Build history of the part. All positions in model axes, mm. A direction names the side the tool comes from. Coordinates: 2 decimals unless noted, no trailing zeros. Order: outer loops, then holes, each group sorted by start corner. A loop starts at its lowest first (then second) coordinate and runs counter-clockwise, first axis right, second up. Notation, with made-up numbers: (-6, 6) - (4, 6) arc R26 ccw to (4, 37) - close; hole circle Ø4 at (-3, 41.5). An arc over 180 degrees is marked (long way). One line per item, written item: value.
from build123d import *

# Parameters (mm, degrees)
SKETCH_1_W          = 13.1
SKETCH_1_H          = 9.245579741
SKETCH_1_R          = 1
EXTRUDE_1_DEPTH     = 1.3
SKETCH_2_W          = 1.5
SKETCH_2_H          = 5
EXTRUDE_2_DEPTH     = 8
SKETCH_4_R          = 1
CUT_EXTRUDE_1_DEPTH = 15


with BuildPart() as part:
    # 草图1 → 凸台-拉伸1 (new body)
    with BuildSketch(Plane.XY):
        with Locations((6.55, 4.622789871)):
            Rectangle(SKETCH_1_W, SKETCH_1_H)
        with Locations((6.55, 7.245579741)):
            Circle(SKETCH_1_R, mode=Mode.SUBTRACT)
    extrude(amount=EXTRUDE_1_DEPTH)

    # 草图2 → 凸台-拉伸2 (add)
    with BuildSketch(Plane.XY.offset(1.3)):
        with Locations((0.75, 2.5)):
            Rectangle(SKETCH_2_W, SKETCH_2_H)
        with Locations((12.35, 2.5)):
            Rectangle(SKETCH_2_W, SKETCH_2_H)
    extrude(amount=EXTRUDE_2_DEPTH)

    # 草图4 → 切除-拉伸1 (cut)
    with BuildSketch(Plane.ZY):
        with Locations((7.3, 2.5)):
            Circle(SKETCH_4_R)
    extrude(amount=-CUT_EXTRUDE_1_DEPTH, mode=Mode.SUBTRACT)


solid = part.part
1. 3-axis set-ups, long thin cutter, end or side, ignore diameter. For faces 4 (the face through (0, 3, 5)), 5 (the face through (1.5, 2, 5)), 6 (the face through (1, 5, 5)): which of +Z, -Z, +X, -X, +Y, -Y reach the whole face in a straight line?
Values found:
face 4: +Z, -Z, -X, +Y, -Y
face 5: +Z, +Y, -Y
face 6: +Z, +X, -X, +Y
2. Flat gauge pins, fed straight in: P1, Ø1.6, axis at x = 12.5, z = 5.5, coming from the +Y side; P2, Ø1, axis at x = 5, y = 2.5, coming from the +Z side; P3, Ø1.2, axis at y = 2.5, z = 7.3, coming from the -X side. Where does each tip first touch, or does it go through?
Values found:
P1: stops at y = 5
P2: stops at z = 1.3
P3: passes through
3. Band-saw the part on B-B, the plane x = 12.25. Give the cut face in (y, z), and give its area (3 significant figures).
Values found:
outline: (0, 0) - (9.25, 0) - (9.25, 1.3) - (5, 1.3) - (5, 9.3) - (0, 9.3) - close; hole circle Ø2 at (2.5, 7.3)
area: 48.9 mm2
4. Band-saw the part on C-C, the plane y = 2.5. Give the cut face in (x, z), and give its area (3 significant figures).
Values found:
outline: (0, 0) - (13.1, 0) - (13.1, 6.3) - (11.6, 6.3) - (11.6, 1.3) - (1.5, 1.3) - (1.5, 6.3) - (0, 6.3) - close; (0, 8.3) - (1.5, 8.3) - (1.5, 9.3) - (0, 9.3) - close; (11.6, 8.3) - (13.1, 8.3) - (13.1, 9.3) - (11.6, 9.3) - close
area: 35.0 mm2
5. Band-saw the part on D-D, the plane x = 6.55. Give the cut face in (y, z), and give its area (3 significant figures).
Values found:
outline: (0, 0) - (6.25, 0) - (6.25, 1.3) - (0, 1.3) - close; (8.25, 0) - (9.25, 0) - (9.25, 1.3) - (8.25, 1.3) - close
area: 9.42 mm2
6. Band-saw the part on A-A, the plane z = 6.5. Give the cut face in (x, y).
Values found:
outline: (0, 0) - (1.5, 0) - (1.5, 1.9) - (0, 1.9) - close; (0, 3.1) - (1.5, 3.1) - (1.5, 5) - (0, 5) - close; (11.6, 0) - (13.1, 0) - (13.1, 1.9) - (11.6, 1.9) - close; (11.6, 3.1) - (13.1, 3.1) - (13.1, 5) - (11.6, 5) - close
7. Two-plate mould, pull along Z, no slides. Class faces 1 (the face through (12, 5, 5)), 2 (the face through (1, 3, 9.3)), 3 (the face through (0.74, 3.49, 7.17)): pulls with the +Z half, pulls with the -Z half, needs draft (parallel to the pull), parting line crosses it, or undercut.
Values found:
face 1: needs draft
face 2: pulls with the +Z half
face 3: undercut
8. Probe line 1 along Y through (x, z) = (0.65, 7.3); line 2 along X through (y, z) = (4.25, 4.5); line 3 along Y through (x, z) = (6.55, 1). List the from-to ranges inside material, lowest first.
Values found:
line 1: y = 0 to 1.5, 3.5 to 5
line 2: x = 0 to 1.5, 11.6 to 13.1
line 3: y = 0 to 6.25, 8.25 to 9.25
